Part model, mm, in its own coordinate system. A direction names the side the tool comes from. Round coordinates to 2 decimals unless told otherwise and drop trailing zeros. Loops run counter-clockwise (first coordinate to the right, second up) from the corner with the lowest first, then second, coordinate; pieces in that order, holes last. Notation, with made-up numbers: (-17, 15) -> (22, 15) arc R30 cw to (22, 51) -> close; hole circle Ø3 at (-19, 83). An arc over 180 degrees is marked (long way). Answer as CSV lines item,"result".
from build123d import *

# Parameters (mm, degrees)
SKETCH1_W                = 10.5
SKETCH1_H                = 20
BOSS_EXTRUDE1_DEPTH      = 10
SHELL2_T                 = -1
SKETCH2_W                = 2.5
SKETCH2_H                = 2.5
CUT_EXTRUDE1_DEPTH       = 1
SKETCH3_W                = 8.5
SKETCH3_H                = 19
CUT_EXTRUDE2_DEPTH       = 1
CUT_EXTRUDE3_DEPTH       = 18.036725037
CUT_EXTRUDE3_DEPTH_BACK  = 18.036725037
SKETCH5_W                = 8.5
SKETCH5_H                = 6.121023644
CUT_EXTRUDE4_DEPTH       = 1
FILLET4_R                = 0.5
CUT_EXTRUDE9_DEPTH       = 17.463595639
CUT_EXTRUDE9_DEPTH_BACK  = 17.463595639
SKETCH10_R               = 0.375
CUT_EXTRUDE10_DEPTH      = 14.182094401
CUT_EXTRUDE10_DEPTH_BACK = 14.182094401
SKETCH11_R               = 0.5


with BuildPart() as part:
    # Sketch1 → Boss-Extrude1 (new body)
    with BuildSketch(Plane(origin=(0, 0, 0), x_dir=(1, 0, 0), z_dir=(0, 1, 0))):
        Rectangle(SKETCH1_W, SKETCH1_H)
    extrude(amount=BOSS_EXTRUDE1_DEPTH)

    # Shell2
    shell2_openings = [part.faces().sort_by_distance(p)[0] for p in [
        (0, 5, 10),
    ]]
    offset(amount=SHELL2_T, openings=shell2_openings, kind=Kind.INTERSECTION)

    # Sketch2 → Cut-Extrude1 (cut)
    with BuildSketch(Plane.XZ):
        with Locations((0, 8.75)):
            Rectangle(SKETCH2_W, SKETCH2_H)
    extrude(amount=-CUT_EXTRUDE1_DEPTH, mode=Mode.SUBTRACT)

    # Sketch3 → Cut-Extrude2 (cut)
    with BuildSketch(Plane.XZ.offset(-9)):
        with Locations((0, 0.5)):
            Rectangle(SKETCH3_W, SKETCH3_H)
    extrude(amount=-CUT_EXTRUDE2_DEPTH, mode=Mode.SUBTRACT)

    # Sketch4 → Cut-Extrude3 (cut, two sides: drawn at the far end of the back side and taken through both)
    with BuildSketch(Plane.ZY.offset(4.25).offset(-CUT_EXTRUDE3_DEPTH_BACK)):
        with BuildLine():
            Line((10, 10), (10, 3.699455157))
            Line((10, 3.699455157), (-6.213436391, 7.674325551))
            ThreePointArc((-6.213436391, 7.674325551), (-8.511231515, 7.441745527), (-10, 5.676094289))
            Line((-10, 5.676094289), (-10, 10))
            Line((-10, 10), (10, 10))
        make_face()
    extrude(amount=CUT_EXTRUDE3_DEPTH + CUT_EXTRUDE3_DEPTH_BACK, mode=Mode.SUBTRACT)

    # Sketch5 → Cut-Extrude4 (cut)
    with BuildSketch(Plane.XY.offset(-9)):
        with Locations((0, 4.060511822)):
            Rectangle(SKETCH5_W, SKETCH5_H)
    extrude(amount=-CUT_EXTRUDE4_DEPTH, mode=Mode.SUBTRACT)

    # Fillet4
    fillet4_edges = [part.edges().sort_by_distance(p)[0] for p in [
        (1.25, 0.5, 10),
        (1.25, 0.5, 7.5),
        (-1.25, 0.5, 7.5),
        (-1.25, 0.5, 10),
    ]]
    fillet(fillet4_edges, radius=FILLET4_R)

    # Sketch10 → Cut-Extrude9 (cut, two sides: drawn at the far end of the back side and taken through both)
    with BuildSketch(Plane.ZY.offset(5.25).offset(-CUT_EXTRUDE9_DEPTH_BACK)):
        with Locations((-7.398050854, 4.796107996)):
            Circle(SKETCH10_R)
    extrude(amount=CUT_EXTRUDE9_DEPTH + CUT_EXTRUDE9_DEPTH_BACK, mode=Mode.SUBTRACT)

    # Sketch11 → Cut-Extrude10 (cut, two sides: drawn at the far end of the back side and taken through both)
    with BuildSketch(Plane(origin=(0, 1, 0), x_dir=(1, 0, 0), z_dir=(0, 1, 0)).offset(-CUT_EXTRUDE10_DEPTH_BACK)):
        with Locations(Location((0, -0.418833411, 0), (0, 0, 270))):
            Circle(SKETCH11_R)
        with Locations(Location((2.767046964, -7.614528741, 0), (0, 0, 270))):
            Circle(SKETCH11_R)
        with Locations(Location((-2.767046964, -7.532135283, 0), (0, 0, 270))):
            Circle(SKETCH11_R)
        with Locations(Location((-2.767046964, 6.776861919, 0), (0, 0, 270))):
            Circle(SKETCH11_R)
        with Locations(Location((2.767046964, 6.776861919, 0), (0, 0, 270))):
            Circle(SKETCH11_R)
    extrude(amount=CUT_EXTRUDE10_DEPTH + CUT_EXTRUDE10_DEPTH_BACK, mode=Mode.SUBTRACT)


solid = part.part
Q1. Two-plate mould, pull along Z, no slides. Class faces 1 (the face through (-2.62, 0.49, 8.01)), 2 (the face through (-2.62, 0.49, -6.3)), 3 (the face through (5.25, 3, 0)), 4 (the face through (-4.74, 7.46, -8.48)): pulls with the +Z half, pulls with the -Z half, needs draft (parallel to the pull), parting line crosses it, or undercut.
Geometry results:
face 1,"undercut"
face 2,"undercut"
face 3,"needs draft"
face 4,"parting line crosses it"
Q2. Drop flat-ended pins along their axis: P1, Ø4, axis at x = 1, z = -2, coming from the +Y side; P2, Ø1.1, axis at x = 0.5, y = 0.5, coming from the +Z side; P3, Ø2, axis at x = -4, z = 0.5, coming from the +Y side. Give the stop position or say it passes through.
Geometry results:
P1,"y = 1"
P2,"z = 7.6"
P3,"y = 6.27"
Q3. Saw through at B-B, the plane y = 4. Write the cut outline in (x, z).
Geometry results:
outline,"(-5.25, -10) -> (-4.25, -10) -> (-4.25, 8.77) -> (-5.25, 8.77) -> close; (4.25, -10) -> (5.25, -10) -> (5.25, 8.77) -> (4.25, 8.77) -> close"
Q4. Which spindle directions (+Z, -Z, +X, -X, +Y, -Y) get a long thin tool onto all of the face, cutting with end or side? Do faces 5 (the face through (1, 1, 0)), 6 (the face through (-5.25, 3, 0)), 7 (the face through (0, 0.5, 7.5)). Say none if no direction does.
Geometry results:
face 5,"+Z, -Z, +Y"
face 6,"+Z, -Z, -X, +Y, -Y"
face 7,"+Z, +Y, -Y"
Q5. Drill centre lines: line 1 along X through (y, z) = (1.75, 0.75); line 2 along Z through (x, y) = (0, 0.35); line 3 along Y through (x, z) = (0.5, 0.75). Where is each one in solid material? Low to high.
Geometry results:
line 1,"-5.25 to -4.25, 4.25 to 5.25"
line 2,"-10 to -0.08, 0.92 to 7.5"
line 3,"0 to 1"
Q6. Saw through at A-A, the plane x = 0. Write the cut outline in (y, z), then the cut area to 3 significant figures.
Geometry results:
outline,"(0, -10) -> (1, -10) -> (1, -0.08) -> (0, -0.08) -> close; (0, 0.92) -> (1, 0.92) -> (1, 7.5) -> (0, 7.5) -> close"
area,"16.5 mm2"
Q7. Saw through at C-C, the plane z = 0.5. Write the cut outline in (x, y).
Geometry results:
outline,"(-5.25, 0) -> (-0.49, 0) -> (-0.49, 1) -> (-4.25, 1) -> (-4.25, 6.03) -> (-5.25, 6.03) -> close; (0.49, 0) -> (5.25, 0) -> (5.25, 6.03) -> (4.25, 6.03) -> (4.25, 1) -> (0.49, 1) -> close"
Q8. Saw through at D-D, the plane x = 3. Write the cut outline in (y, z), then the cut area to 3 significant figures.
Geometry results:
outline,"(0, -10) -> (1, -10) -> (1, -7.22) -> (0, -7.22) -> close; (0, -6.33) -> (1, -6.33) -> (1, 7.17) -> (0, 7.17) -> close; (0, 8.06) -> (1, 8.06) -> (1, 10) -> (0, 10) -> close"
area,"18.2 mm2"
